Part model, mm, in its own coordinate system. A direction names the side the tool comes from. Coordinates: 2 decimals unless noted, no trailing zeros. Write each loop counter-clockwise with the first axis right and the second up, starting at its lowest first coordinate (ties: lowest second). Pieces come first, ordered by that corner, then holes. Notation, with made-up numbers: (88.25, 6.25) -> (128.25, 6.25) arc R7 cw to (128.25, 14.25) -> close; hole circle Ø8 at (50, 88.25). An arc over 180 degrees is marked (long way). Write item = value, one per line.
from build123d import *

# Parameters (mm, degrees)
F1_DEPTH = 570
F3_DEPTH = 50
F5_DEPTH = 50


# Not quite as in the source:
# - a feature names something its author has since deleted; it is built from what else it names


with BuildPart() as f1:
    # F0 (on Front) → F1 (new body, symmetric)
    with BuildSketch(Plane.XZ):
        Polygon((0, 50), (0, 0), (50, 0), (50, 5), (5, 5), (5, 50), align=None)
    extrude(amount=F1_DEPTH, both=True)

    # F2 (on face) → F3 (cut)
    with BuildSketch(Plane(origin=(0, 0, 0), x_dir=(0, -1, 0), z_dir=(-1, 0, 0))):
        Polygon((-570, 50), (-570, 0), (-520, 50), align=None)
        Polygon((520, 50), (570, 0), (570, 50), align=None)
    extrude(amount=-F3_DEPTH, mode=Mode.SUBTRACT)

    # F4 (on face) → F5 (cut)
    with BuildSketch(Plane(origin=(0, 0, 0), x_dir=(1, 0, 0), z_dir=(0, 0, -1))):
        Polygon((50, -520), (0, -570), (50, -570), align=None)
    extrude(amount=-F5_DEPTH, mode=Mode.SUBTRACT)


solid = f1.part
Q1. Pin check, flat tips, straight feed: pin 1 (12 mm diameter, centred on y = 297.5, z = 19.5, fed in from +X); pin 2 (1.5 mm diameter, centred on x = 33.5, y = -83.5, fed in from +Z). Stop position of each tip, or through.
Model answer:
pin_1 = 5
pin_2 = 5
Q2. Saw through at B-B on z = 40. Give the cut face in (x, y).
Model answer:
outline = (0, -530) -> (5, -530) -> (5, 530) -> (0, 530) -> close
Q3. Probe line 1 (X direction, y = 108, z = 33); line 2 (Y direction, x = 12, z = 3). List the from-to ranges inside material, lowest first. Write a range as from..to.
Model answer:
line_1 = 0..5
line_2 = -567..558
Q4. Which spindle directions (+Z, -Z, +X, -X, +Y, -Y) get a long thin tool onto all of the face, cutting with end or side? Do faces 1 (the face through (28, -8, 5)), 2 (the face through (0, -8, 25)). Say none if no direction does.
Model answer:
face_1 = +Z, +X, +Y, -Y
face_2 = +Z, -Z, -X, +Y, -Y
Q5. Saw through at A-A on x = 13. Give the cut face in (y, z), and give its area (3 significant figures).
Model answer:
outline = (-570, 0) -> (557, 0) -> (557, 5) -> (-565, 5) -> close
area = 5,620 mm²
Q6. Saw through at C-C on y = 161. Give the cut face in (x, z).
Model answer:
outline = (0, 0) -> (50, 0) -> (50, 5) -> (5, 5) -> (5, 50) -> (0, 50) -> close
